```python
from build123d import *

# Parameters (mm, degrees)
SKETCH1_W           = 73.025
SKETCH1_H           = 73.025
BOSS_EXTRUDE1_DEPTH = 12.7
SKETCH2_R           = 3.175
CUT_EXTRUDE1_DEPTH  = 3.175
SKETCH3_R           = 4.7625
CUT_EXTRUDE2_DEPTH  = 10.525
CHAMFER1_SIZE       = 6.35


with BuildPart() as part:
    # Sketch1 → Boss-Extrude1 (new body)
    with BuildSketch(Plane.XY):
        Rectangle(SKETCH1_W, SKETCH1_H)
    extrude(amount=-BOSS_EXTRUDE1_DEPTH)

    # Sketch2 → Cut-Extrude1 (cut)
    with BuildSketch(Plane.XY):
        Circle(SKETCH2_R)
    extrude(amount=-CUT_EXTRUDE1_DEPTH, mode=Mode.SUBTRACT)

    # Sketch3 → Cut-Extrude2 (cut, through all)
    with BuildSketch(Plane.XY.offset(-3.175)):
        Circle(SKETCH3_R)
    extrude(amount=-CUT_EXTRUDE2_DEPTH, mode=Mode.SUBTRACT)

    # Chamfer1
    chamfer1_edges = [part.edges().sort_by_distance(p)[0] for p in [
        (0, 36.5125, 0),
        (36.5125, 0, 0),
        (0, -36.5125, 0),
        (-36.5125, 0, 0),
    ]]
    chamfer(chamfer1_edges, length=CHAMFER1_SIZE)


solid = part.part
```
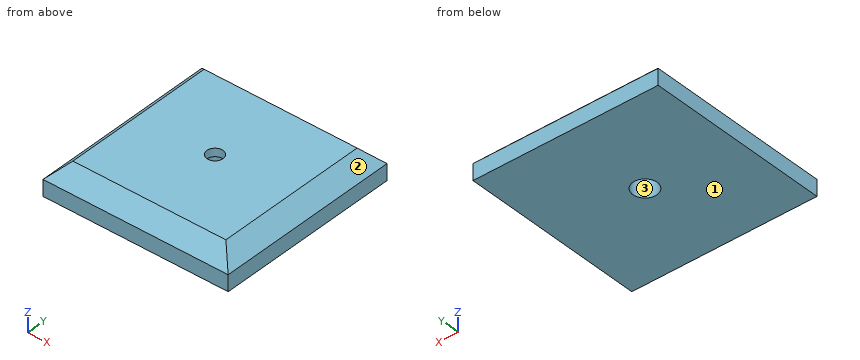
For this review, take the finished solid that the model builds, in its own axes (mm). Face numbers are marked on the shaded views. Coordinates: 2 decimals unless noted, no trailing zeros. Loops run counter-clockwise (first coordinate to the right, second up) from the corner with the lowest first, then second, coordinate; pieces in that order, holes last. Notation, with made-up numbers: (-28, 38) -> (11, 38) arc R7 ccw to (11, 47) -> close; hole circle Ø1 at (51.5, -33.5). An arc over 180 degrees is marked (long way). Return JSON: item names as keys, results as strings. Group by question number.
(1) Mouldability with a two-part tool opening along X and no side actions: class the marked faces 1, 2 and 3 as pulls with the +X half, pulls with the -X half, needs draft (parallel to the pull), parting line crosses it, or undercut.
(2) For pin 1 Ø5 at (x, y) = (-0.5, -2) entering from -Z (3 decimals), flat-tipped, find the tip position at first contact; note if it passes through.
(3) To check wall thickness, follow L1, parallel to Y at x = 0, z = -11; L2, parallel to Y at x = 0, z = -1.15 (1 decimal); L3, parallel to Z at x = 33, y = -20.5. State the ranges of each line that lie inside material, in increasing order.
(4) Consider section C-C, the plane x = 17. Give the boundary of the cut face in (y, z), plus the area to 3 significant figures.
Results below:
{
 "1": {"face 1": "needs draft", "face 2": "pulls with the +X half", "face 3": "undercut"},
 "2": {"pin 1": "stops at z = -3.175"},
 "3": {"L1": "y = -36.51 to -4.76, 4.76 to 36.51", "L2": "y = -31.3 to -3.2, 3.2 to 31.3", "L3": "z = -12.7 to -2.84"},
 "4": {"outline": "(-36.51, -12.7) -> (36.51, -12.7) -> (36.51, -6.35) -> (30.16, 0) -> (-30.16, 0) -> (-36.51, -6.35) -> close", "area": "887 mm2"}
}
